```python
from build123d import *

# Parameters (mm, degrees)
SKETCH2_W           = 220
SKETCH2_H           = 220
BOSS_EXTRUDE1_DEPTH = 6
FILLET1_R           = 10
BOSS_EXTRUDE3_DEPTH = 53
BOSS_EXTRUDE4_START = 22
BOSS_EXTRUDE4_DEPTH = 22
FILLET2_R           = 2
CUT_EXTRUDE2_REACH  = 168.376
SKETCH7_R           = 10
CUT_EXTRUDE3_REACH  = 168.376
SKETCH8_R           = 1.6


with BuildPart() as part:
    # Sketch2 → Boss-Extrude1 (new body)
    with BuildSketch(Plane(origin=(0, 0, 0), x_dir=(1, 0, 0), z_dir=(0, 1, 0))):
        Rectangle(SKETCH2_W, SKETCH2_H)
    extrude(amount=BOSS_EXTRUDE1_DEPTH)

    # Fillet1
    fillet1_edges = [part.edges().sort_by_distance(p)[0] for p in [
        (110, 3, 110),
        (-110, 3, 110),
        (-110, 3, -110),
        (110, 3, -110),
    ]]
    fillet(fillet1_edges, radius=FILLET1_R)

    # Sketch4 → Boss-Extrude3 (add)
    with BuildSketch(Plane(origin=(0, 6, 0), x_dir=(1, 0, 0), z_dir=(0, 1, 0))):
        with BuildLine():
            ThreePointArc((-105.325, -85), (-99.371945328, -99.371945328), (-85, -105.325))
            ThreePointArc((-85, -105.325), (-82.675, -103), (-85, -100.675))
            ThreePointArc((-85, -100.675), (-96.083898795, -96.083898795), (-100.675, -85))
            ThreePointArc((-100.675, -85), (-103, -82.675), (-105.325, -85))
        make_face()
        with BuildLine():
            ThreePointArc((106.325, -85), (100.079052109, -100.079052109), (85, -106.325))
            ThreePointArc((85, -106.325), (81.675, -103), (85, -99.675))
            ThreePointArc((85, -99.675), (95.376792014, -95.376792014), (99.675, -85))
            ThreePointArc((99.675, -85), (103, -81.675), (106.325, -85))
        make_face()
        with BuildLine():
            ThreePointArc((106.325, 85), (100.079052109, 100.079052109), (85, 106.325))
            ThreePointArc((85, 106.325), (81.675, 103), (85, 99.675))
            ThreePointArc((85, 99.675), (95.376792014, 95.376792014), (99.675, 85))
            ThreePointArc((99.675, 85), (103, 81.675), (106.325, 85))
        make_face()
        with BuildLine():
            ThreePointArc((-106.325, 85), (-100.079052109, 100.079052109), (-85, 106.325))
            ThreePointArc((-85, 106.325), (-81.675, 103), (-85, 99.675))
            ThreePointArc((-85, 99.675), (-95.376792014, 95.376792014), (-99.675, 85))
            ThreePointArc((-99.675, 85), (-103, 81.675), (-106.325, 85))
        make_face()
    extrude(amount=BOSS_EXTRUDE3_DEPTH)

    # Sketch3 → Boss-Extrude4 (add)
    with BuildSketch(Plane(origin=(0, 6, 0), x_dir=(1, 0, 0), z_dir=(0, 1, 0)).offset(BOSS_EXTRUDE4_START)):
        with BuildLine():
            Line((75, 95), (75, 110))
            Line((75, 110), (100, 110))
            ThreePointArc((100, 110), (107.071067812, 107.071067812), (110, 100))
            Line((110, 100), (110, 75))
            Line((110, 75), (95, 75))
            Line((95, 75), (95, 85))
            ThreePointArc((95, 85), (92.071067812, 92.071067812), (85, 95))
            Line((85, 95), (75, 95))
        make_face()
        with BuildLine():
            Line((-75, 110), (-100, 110))
            ThreePointArc((-100, 110), (-107.071067812, 107.071067812), (-110, 100))
            Line((-110, 100), (-110, 75))
            Line((-110, 75), (-95, 75))
            Line((-95, 75), (-95, 85))
            ThreePointArc((-95, 85), (-92.071067812, 92.071067812), (-85, 95))
            Line((-85, 95), (-75, 95))
            Line((-75, 95), (-75, 110))
        make_face()
        with BuildLine():
            Line((-75, -95), (-75, -110))
            Line((-75, -110), (-100, -110))
            ThreePointArc((-100, -110), (-107.071067812, -107.071067812), (-110, -100))
            Line((-110, -100), (-110, -75))
            Line((-110, -75), (-95, -75))
            Line((-95, -75), (-95, -85))
            ThreePointArc((-95, -85), (-92.071067812, -92.071067812), (-85, -95))
            Line((-85, -95), (-75, -95))
        make_face()
        with BuildLine():
            Line((75, -110), (100, -110))
            ThreePointArc((100, -110), (107.071067812, -107.071067812), (110, -100))
            Line((110, -100), (110, -75))
            Line((110, -75), (95, -75))
            Line((95, -75), (95, -85))
            ThreePointArc((95, -85), (92.071067812, -92.071067812), (85, -95))
            Line((85, -95), (75, -95))
            Line((75, -95), (75, -110))
        make_face()
    extrude(amount=-BOSS_EXTRUDE4_DEPTH)

    # Fillet2
    fillet2_edges = [part.edges().sort_by_distance(p)[0] for p in [
        (75, 17, -95),
        (95, 17, -75),
        (110, 17, -75),
        (75, 17, -110),
        (-110, 17, -75),
        (-95, 17, -75),
        (-75, 17, -95),
        (-75, 17, -110),
        (-95, 17, 75),
        (-110, 17, 75),
        (-75, 17, 110),
        (-75, 17, 95),
        (110, 17, 75),
        (95, 17, 75),
        (75, 17, 95),
        (75, 17, 110),
    ]]
    fillet(fillet2_edges, radius=FILLET2_R)

    # Sketch7 → Cut-Extrude2 (cut, up to next)
    with BuildSketch(Plane.XZ, mode=Mode.PRIVATE) as cut_extrude2_sk1:
        with Locations(Location((30, 0, 0), (0, 0, 270))):
            Circle(SKETCH7_R)
    cut_extrude2_tool1 = extrude(cut_extrude2_sk1.sketch, amount=-CUT_EXTRUDE2_REACH, mode=Mode.PRIVATE) & part.part
    add(cut_extrude2_tool1.solids().sort_by_distance((30, 0, 0))[0], mode=Mode.SUBTRACT)

    # Sketch8 → Cut-Extrude3 (cut, up to next)
    with BuildSketch(Plane.XZ, mode=Mode.PRIVATE) as cut_extrude3_sk1:
        with Locations(Location((-104, 10, 0), (0, 0, 270))):
            Circle(SKETCH8_R)
    cut_extrude3_tool1 = extrude(cut_extrude3_sk1.sketch, amount=-CUT_EXTRUDE3_REACH, mode=Mode.PRIVATE) & part.part
    # Sketch8 → Cut-Extrude3 (cut, up to next)
    with BuildSketch(Plane.XZ, mode=Mode.PRIVATE) as cut_extrude3_sk2:
        with Locations(Location((-104, -10, 0), (0, 0, 270))):
            Circle(SKETCH8_R)
    cut_extrude3_tool2 = extrude(cut_extrude3_sk2.sketch, amount=-CUT_EXTRUDE3_REACH, mode=Mode.PRIVATE) & part.part
    # Sketch8 → Cut-Extrude3 (cut, up to next)
    with BuildSketch(Plane.XZ, mode=Mode.PRIVATE) as cut_extrude3_sk3:
        with Locations(Location((-10, 104, 0), (0, 0, 270))):
            Circle(SKETCH8_R)
    cut_extrude3_tool3 = extrude(cut_extrude3_sk3.sketch, amount=-CUT_EXTRUDE3_REACH, mode=Mode.PRIVATE) & part.part
    # Sketch8 → Cut-Extrude3 (cut, up to next)
    with BuildSketch(Plane.XZ, mode=Mode.PRIVATE) as cut_extrude3_sk4:
        with Locations(Location((10, 104, 0), (0, 0, 270))):
            Circle(SKETCH8_R)
    cut_extrude3_tool4 = extrude(cut_extrude3_sk4.sketch, amount=-CUT_EXTRUDE3_REACH, mode=Mode.PRIVATE) & part.part
    # Sketch8 → Cut-Extrude3 (cut, up to next)
    with BuildSketch(Plane.XZ, mode=Mode.PRIVATE) as cut_extrude3_sk5:
        with Locations(Location((104, 10, 0), (0, 0, 270))):
            Circle(SKETCH8_R)
    cut_extrude3_tool5 = extrude(cut_extrude3_sk5.sketch, amount=-CUT_EXTRUDE3_REACH, mode=Mode.PRIVATE) & part.part
    # Sketch8 → Cut-Extrude3 (cut, up to next)
    with BuildSketch(Plane.XZ, mode=Mode.PRIVATE) as cut_extrude3_sk6:
        with Locations(Location((104, -10, 0), (0, 0, 270))):
            Circle(SKETCH8_R)
    cut_extrude3_tool6 = extrude(cut_extrude3_sk6.sketch, amount=-CUT_EXTRUDE3_REACH, mode=Mode.PRIVATE) & part.part
    # Sketch8 → Cut-Extrude3 (cut, up to next)
    with BuildSketch(Plane.XZ, mode=Mode.PRIVATE) as cut_extrude3_sk7:
        with Locations(Location((10, -104, 0), (0, 0, 270))):
            Circle(SKETCH8_R)
    cut_extrude3_tool7 = extrude(cut_extrude3_sk7.sketch, amount=-CUT_EXTRUDE3_REACH, mode=Mode.PRIVATE) & part.part
    # Sketch8 → Cut-Extrude3 (cut, up to next)
    with BuildSketch(Plane.XZ, mode=Mode.PRIVATE) as cut_extrude3_sk8:
        with Locations(Location((-10, -104, 0), (0, 0, 270))):
            Circle(SKETCH8_R)
    cut_extrude3_tool8 = extrude(cut_extrude3_sk8.sketch, amount=-CUT_EXTRUDE3_REACH, mode=Mode.PRIVATE) & part.part
    add(cut_extrude3_tool1.solids().sort_by_distance((-104, 0, 10))[0], mode=Mode.SUBTRACT)
    add(cut_extrude3_tool2.solids().sort_by_distance((-104, 0, -10))[0], mode=Mode.SUBTRACT)
    add(cut_extrude3_tool3.solids().sort_by_distance((-10, 0, 104))[0], mode=Mode.SUBTRACT)
    add(cut_extrude3_tool4.solids().sort_by_distance((10, 0, 104))[0], mode=Mode.SUBTRACT)
    add(cut_extrude3_tool5.solids().sort_by_distance((104, 0, 10))[0], mode=Mode.SUBTRACT)
    add(cut_extrude3_tool6.solids().sort_by_distance((104, 0, -10))[0], mode=Mode.SUBTRACT)
    add(cut_extrude3_tool7.solids().sort_by_distance((10, 0, -104))[0], mode=Mode.SUBTRACT)
    add(cut_extrude3_tool8.solids().sort_by_distance((-10, 0, -104))[0], mode=Mode.SUBTRACT)


solid = part.part
```
Can you work these out from the model? Positions are in its coordinate system, mm. A direction names the side the tool comes from. Give positions to 0.01 mm unless a question says otherwise; leave off trailing zeros. Loops run counter-clockwise (first coordinate to the right, second up) from the corner with the lowest first, then second, coordinate; pieces in that order, holes last. Notation, with made-up numbers: M 18,39.25 L 60,39.25 A25 ccw 60,62.25 Z; hole C -35,84.25 d6. An arc over 180 degrees is marked long. Use one line per item in the form item = value. Start each with the question number.
(1) I want a section at D-D, the plane z = -62. Write out the boundary of the cut face in (x, y).
(2) I want a section at C-C, the plane z = 2.5. Write out the boundary of the cut face in (x, y), and give its area (3 significant figures).
(3) I want a section at A-A, the plane y = 48.5. Write out the boundary of the cut face in (x, z) (3 decimals), and give its area (3 significant figures).
(4) I'm going to push flat-ended pins straight in: P1, Ø5.5, axis at x = 103.5, y = 17, coming from the +Z side; P2, Ø10.5, axis at x = 92.5, z = 90.5, coming from the +Y side; P3, Ø3, axis at x = 82.5, z = 80.5, coming from the +Y side. Where does each tip first touch, or does it pass through?
(5) Thinking about a two-plate mould opening in X: for faces 4 (the flat face through (-103, 17, -75)), 5 (the cylindrical face through (95.26, 43.28, 95.49)), which applies, released by +X, released by -X, zero draft, split by the parting line, or undercut?
(6) Please list where these lines run through material, in increasing order: line 1 (Z direction, x = 83, y = 12); line 2 (Z direction, x = -104, y = 4.65); line 3 (Y direction, x = -29.5, z = -56.5).
(7) I want a section at B-B, the plane x = 30. Write out the boundary of the cut face in (y, z).
(8) On a 3-axis mill with a long thin cutter (end or side, diameter ignored), from which of +Z, -Z, +X, -X, +Y, -Y can I reach the whole of each face in a straight line? I mean faces 1 (the flat face through (-75, 17, -102)), 2 (the flat face through (103, 17, -75)), 3 (the flat face through (96, 28, 92)). Say none if no direction works.
Worked out:
q1.outline = M -110,0 L 110,0 L 110,6 L -110,6 Z
q2.outline = M -110,0 L 20.32,0 L 20.32,6 L -110,6 Z; M 39.68,0 L 110,0 L 110,6 L 39.68,6 Z
q2.area = 1,200 mm²
q3.outline = M -106.325,-85 A21.325 ccw -85,-106.325 A3.325 ccw -85,-99.675 A14.675 cw -99.675,-85 A3.325 ccw Z; M -105.325,85 A2.325 ccw -100.675,85 A15.675 cw -85,100.675 A2.325 ccw -85,105.325 A20.325 ccw Z; M 85,-106.325 A21.325 ccw 106.325,-85 A3.325 ccw 99.675,-85 A14.675 cw 85,-99.675 A3.325 ccw Z; M 85,99.675 A14.675 cw 99.675,85 A3.325 ccw 106.325,85 A21.325 ccw 85,106.325 A3.325 ccw Z
q3.area = 817 mm²
q4.P1 = 109.97
q4.P2 = 28
q4.P3 = 6
q5.face_4 = zero draft
q5.face_5 = undercut
q6.line_1 = -110 to -95, 95 to 110
q6.line_2 = -109.17 to -11.6, -8.4 to 8.4, 11.6 to 109.17
q6.line_3 = 0 to 6
q7.outline = M 0,-110 L 6,-110 L 6,-10 L 0,-10 Z; M 0,10 L 6,10 L 6,110 L 0,110 Z
q8.face_1 = +Z, -Z, +Y
q8.face_2 = +X, -X, +Y
q8.face_3 = +Y
